Autodesk Fusion 360 part; units mm, degrees
sketch "Sketch1" plane through (0, 0, 0) normal (0, 0, 1) x (1, 0, 0)
  circle A0 centre (0, 0) radius 12.7
  circle A1 centre (0, 0) radius 5.08
  dimension "d1" = 25.4
  dimension "d3" = 10.16
extrude "Extrude1" add sketch "Sketch1" along normal blind 6.35
sketch "Sketch3" plane through (0, 0, 6.35) normal (0, 0, 1) x (-1, 0, 0)
  circle A0 centre (0, 0) radius 5.08
  circle A1 centre (0, 0) radius 12.7
  line L0 (0, 5.08) -> (0, 12.7)
  circle A2 centre (0, 0) radius 8.89
  point P0 (0, 8.89)
hole "Hole1" at (0, -8.89, 6.35) direction (0, 0, -1) diameter 3.175 depth 6.35 tip angle 180 counterbore diameter 5.08 counterbore depth 2.54
pattern_circular "C-Pattern1" count 6 over 360 about axis through (0, 0, 0) along (0, 0, 1) of "Hole1"
fillet "Fillet1" radius 0.635 2 edges at (-11.8406, -4.5925, 6.35) (-11.8406, -4.5925, 0)
Design review of the part built by this model. Coordinates are the model's own, in mm. A direction names the side the tool comes from. Give positions to 0.01 mm unless a question says otherwise; leave off trailing zeros. Write each loop counter-clockwise with the first axis right and the second up, starting at its lowest first coordinate (ties: lowest second). Pieces come first, ordered by that corner, then holes. Notation, with made-up numbers: M 61.25,61 L 113.25,61 A10 ccw 113.25,76 Z; hole C -33.5,33 d8. An arc over 180 degrees is marked long. Answer as a JSON object with one key per item and string values. Group by question number.
1) Tool access review of faces 1 (the face through (1.546, -6.874, 5.062)), 2 (the face through (8.665, 5.705, 1.878)): name each direction out of +Z, -Z, +X, -X, +Y, -Y from which nothing blocks a thin tool from reaching the whole face with its end or side.
2) We need section B-B (z = 4.5). Give the boundary of the cut face in (x, y) (3 decimals), and give its area (3 significant figures).
3) We need section C-C (y = -4.25). Count the separate pieces of the cut face and the enclosed holes in it, and give its area (3 significant figures).
4) For line 1 along Y through (x, z) = (-2.25, 4); line 2 along Y through (x, z) = (-7, 4); line 3 along X through (y, z) = (-3.5, 1), list the stretches that pass through material, from the lowest coordinate up.
5) We need section A-A (y = 0). Give the boundary of the cut face in (x, z) (3 decimals), and give its area (3 significant figures).
6) Mouldability with a two-part tool opening along X and no side actions: class faces 3 (the face through (-8.665, -5.705, 1.878)), 4 (the face through (5, -3, 0)) as released by +X, released by -X, zero draft, split by the parting line, or undercut.
7) Clearance check with flat-ended pins moving along their axes: pin 1 Ø3 at (x, y) = (7.5, -7) entering from -Z; pin 2 Ø1.5 at (x, y) = (6.5, -5) entering from +Z; pin 3 Ø1.5 at (x, z) = (-8, 2.5) entering from -Y; pin 4 Ø1 at (x, z) = (4.5, 2) entering from -Y. State where each tip first meets the part, or that it passes through.
Answer key:
{
 "1": {"face 1": "+Z", "face 2": "+Z, -Z"},
 "2": {"outline": "C 0,0 d25.4; hole C -7.699,-4.445 d5.08; hole C -7.699,4.445 d5.08; hole C 0,0 d10.16; hole C 0,-8.89 d5.08; hole C 0,8.89 d5.08; hole C 7.699,-4.445 d5.08; hole C 7.699,4.445 d5.08", "area": "304 mm²"},
 "3": {"separate pieces": "4", "enclosed holes": "0", "area": "66.5 mm²"},
 "4": {"line 1": "y = -12.5 to -10.07, -7.71 to -4.55, 4.55 to 7.71, 10.07 to 12.5", "line 2": "y = -10.6 to -6.89, -2 to 2, 6.89 to 10.6", "line 3": "x = -12.21 to -8.97, -6.42 to -3.68, 3.68 to 6.42, 8.97 to 12.21"},
 "5": {"outline": "M -12.7,0.635 A0.635 ccw -12.065,0 L -5.08,0 L -5.08,6.35 L -12.065,6.35 A0.635 ccw -12.7,5.715 Z; M 5.08,0 L 12.065,0 A0.635 ccw 12.7,0.635 L 12.7,5.715 A0.635 ccw 12.065,6.35 L 5.08,6.35 Z", "area": "96.4 mm²"},
 "6": {"face 3": "undercut", "face 4": "zero draft"},
 "7": {"pin 1": "stops at z = 0", "pin 2": "stops at z = 3.81", "pin 3": "stops at y = -10.43", "pin 4": "stops at y = -12.05"}
}
